from build123d import *

# Parameters (mm, degrees)
SKETCH1_W               = 673.1
SKETCH1_H               = 444.5
BOSS_EXTRUDE1_DEPTH     = 7.9375
SKETCH2_W               = 601.6625
SKETCH2_H               = 341.3125
CUT_EXTRUDE1_DEPTH      = 1
CUT_EXTRUDE1_DEPTH_BACK = 16.875
SKETCH8_W               = 601.6625
SKETCH8_H               = 341.3125
SKETCH8_W_2             = 550.8625
SKETCH8_H_2             = 290.5125
BOSS_EXTRUDE3_DEPTH     = 2.54


with BuildPart() as part:
    # Sketch1 → Boss-Extrude1 (new body, symmetric)
    with BuildSketch(Plane.XY):
        Rectangle(SKETCH1_W, SKETCH1_H)
    extrude(amount=BOSS_EXTRUDE1_DEPTH, both=True)

    # Sketch2 → Cut-Extrude1 (cut, two sides)
    with BuildSketch(Plane.XY.offset(7.9375)) as cut_extrude1_sk:
        Rectangle(SKETCH2_W, SKETCH2_H)
    extrude(amount=CUT_EXTRUDE1_DEPTH, mode=Mode.SUBTRACT)
    extrude(cut_extrude1_sk.sketch, amount=-CUT_EXTRUDE1_DEPTH_BACK, mode=Mode.SUBTRACT)

    # Sketch8 → Boss-Extrude3 (add)
    with BuildSketch(Plane.XY.offset(7.9375)):
        Rectangle(SKETCH8_W, SKETCH8_H)
        Rectangle(SKETCH8_W_2, SKETCH8_H_2, mode=Mode.SUBTRACT)
    extrude(amount=-BOSS_EXTRUDE3_DEPTH)


solid = part.part
Work out the finished part from the listing and answer in its coordinate system (mm). A direction names the side the tool comes from. Coordinates: 2 decimals unless noted, no trailing zeros. Write each loop counter-clockwise with the first axis right and the second up, starting at its lowest first coordinate (ties: lowest second). Pieces come first, ordered by that corner, then holes. Notation, with made-up numbers: (84, 84) - (98, 84) arc R29 cw to (98, 122) - close; hole circle Ø3 at (-12, 81). An arc over 180 degrees is marked (long way). One line per question, with ' | ' between items.
1) Consider probe 1 along X at (y, z) = (-55, -1); probe 2 along Y at (x, z) = (-291, -6.5); probe 3 along X at (y, z) = (81.5, 6.5). Determine where each line is inside the solid, lowest interval first. Write a range as [from, to].
Checks:
probe 1: [-336.55, -300.83], [300.83, 336.55] | probe 2: [-222.25, -170.66], [170.66, 222.25] | probe 3: [-336.55, -275.43], [275.43, 336.55]
2) For faces 1 (the face through (-4, 170.656, -1)), 2 (the face through (-5, -222.25, 0)), determine the directions among +Z, -Z, +X, -X, +Y, -Y from which every point of the face is accessible in a straight line to the end or side of a thin tool.
Checks:
face 1: -Z | face 2: +Z, -Z, +X, -X, -Y
3) The mould has two halves that part along Y. Classify faces 3 (the face through (-27, -180, -7.938)), 4 (the face through (-24, -151, 5.398)), 5 (the face through (-5, 222.25, 0)): +Y half, -Y half, draft (parallel to the pull), parting line (faces both ways), or undercut.
Checks:
face 3: draft | face 4: undercut | face 5: +Y half
4) Find section C-C, the plane y = 116. Determine the outline of the cut face in (x, z).
Checks:
outline: (-336.55, -7.94) - (-300.83, -7.94) - (-300.83, 5.4) - (-275.43, 5.4) - (-275.43, 7.94) - (-336.55, 7.94) - close; (275.43, 5.4) - (300.83, 5.4) - (300.83, -7.94) - (336.55, -7.94) - (336.55, 7.94) - (275.43, 7.94) - close
5) Find section B-B, the plane z = -3. Determine the outline of the cut face in (x, y), and give its area (3 significant figures).
Checks:
outline: (-336.55, -222.25) - (336.55, -222.25) - (336.55, 222.25) - (-336.55, 222.25) - close; hole (-300.83, -170.66) - (300.83, -170.66) - (300.83, 170.66) - (-300.83, 170.66) - close | area: 93,800 mm2
6) Find section A-A, the plane x = -23.5. Determine the outline of the cut face in (y, z), and give its area (3 significant figures).
Checks:
outline: (-222.25, -7.94) - (-170.66, -7.94) - (-170.66, 5.4) - (-145.26, 5.4) - (-145.26, 7.94) - (-222.25, 7.94) - close; (145.26, 5.4) - (170.66, 5.4) - (170.66, -7.94) - (222.25, -7.94) - (222.25, 7.94) - (145.26, 7.94) - close | area: 1,770 mm2
